Can you work these out from the model? Positions are in its coordinate system, mm. A direction names the side the tool comes from. Round coordinates to 2 decimals unless told otherwise and drop trailing zeros. Loops run counter-clockwise (first coordinate to the right, second up) from the corner with the lowest first, then second, coordinate; pieces in that order, holes last. Notation, with made-up numbers: (49.25, 72.5) -> (74.25, 72.5) arc R21 cw to (74.25, 108.5) -> close; hole circle Ø1 at (22, 65.25). An arc over 180 degrees is marked (long way). Write item = value, one per line.
from build123d import *

# Parameters (mm, degrees)
ESTRUSIONE_ESTRUSIONE1_DEPTH   = 23
FORO_PER_VITE_M3_1_D           = 3.4
FORO_PER_VITE_M3_1_DEPTH       = 34
FORO_PER_VITE_M3_1_CSINK_D     = 3.45
FORO_PER_VITE_M3_1_CSINK_ANGLE = 90
FORO_PER_VITE_M3_1_TIP         = 1.021463052
SCHIZZO5_R                     = 11
ESTRUSIONE_ESTRUSIONE2_DEPTH   = 2
SCHIZZO6_R                     = 2.5
ESTRUSIONE_ESTRUSIONE3_DEPTH   = 18
TAGLIO_ESTRUSIONE1_START       = -17
TAGLIO_ESTRUSIONE1_DEPTH       = 17


with BuildPart() as part:
    # Schizzo1 → Estrusione-Estrusione1 (new body)
    with BuildSketch(Plane(origin=(0, 0, 0), x_dir=(1, 0, 0), z_dir=(0, 1, 0))):
        Polygon((21.15, -17.15), (21.15, 17.15), (17.15, 21.15), (-17.15, 21.15), (-21.15, 17.15), (-21.15, -17.15), (-17.15, -21.15), (17.15, -21.15), align=None)
    extrude(amount=ESTRUSIONE_ESTRUSIONE1_DEPTH)

    # Foro per Vite M3-1
    with Locations(Plane(origin=(0, 0, 0), x_dir=(-1, 0, 0), z_dir=(0, -1, 0))):
        with Locations((-15.5, 15.5), (15.5, 15.5), (15.5, -15.5), (-15.5, -15.5)):
            CounterSinkHole(FORO_PER_VITE_M3_1_D / 2, FORO_PER_VITE_M3_1_CSINK_D / 2, depth=FORO_PER_VITE_M3_1_DEPTH, counter_sink_angle=FORO_PER_VITE_M3_1_CSINK_ANGLE)
            with Locations((0, 0, -(FORO_PER_VITE_M3_1_DEPTH + FORO_PER_VITE_M3_1_TIP / 2))):  # 118° drill point
                Cone(0, FORO_PER_VITE_M3_1_D / 2, FORO_PER_VITE_M3_1_TIP, mode=Mode.SUBTRACT)

    # Schizzo5 → Estrusione-Estrusione2 (add)
    with BuildSketch(Plane(origin=(0, 23, 0), x_dir=(1, 0, 0), z_dir=(0, 1, 0))):
        with Locations(Location((0, 0, 0), (0, 0, 270))):
            Circle(SCHIZZO5_R)
    extrude(amount=ESTRUSIONE_ESTRUSIONE2_DEPTH)

    # Schizzo6 → Estrusione-Estrusione3 (add)
    with BuildSketch(Plane(origin=(0, 25, 0), x_dir=(1, 0, 0), z_dir=(0, 1, 0))):
        with Locations(Location((0, 0, 0), (0, 0, 270))):
            Circle(SCHIZZO6_R)
    extrude(amount=ESTRUSIONE_ESTRUSIONE3_DEPTH)

    # Schizzo7 → Taglio-Estrusione1 (cut)
    with BuildSketch(Plane(origin=(0, 43, 0), x_dir=(1, 0, 0), z_dir=(0, 1, 0)).offset(TAGLIO_ESTRUSIONE1_START)):
        with BuildLine():
            Line((-1.5, 2), (1.5, 2))
            ThreePointArc((1.5, 2), (0, 2.5), (-1.5, 2))
        make_face()
    extrude(amount=TAGLIO_ESTRUSIONE1_DEPTH, mode=Mode.SUBTRACT)


solid = part.part
1. I need wall thicknesses on line 1 (X direction, y = 8.5, z = -15.5); line 2 (Z direction, x = 15, y = 5). Which ranges of each line are inside material? Lowest first, please. Write a range as [from, to].
Entries:
line_1 = [-21.15, -17.2], [-13.8, 13.8], [17.2, 21.15]
line_2 = [-21.15, -17.12], [-13.88, 13.88], [17.12, 21.15]
2. For faces 4 (the flat face through (0, 34, -2)), 5 (the cylindrical face through (0.751, 33.874, 2.385)), 6 (the cylindrical face through (-14.7, 11.7, -14)), which set-ups out of +Z, -Z, +X, -X, +Y, -Y let a thin tool reach every point of the face, with its end or its side?
Entries:
face_4 = -Z, +X, -X, +Y
face_5 = +Y
face_6 = +Y, -Y
3. I'm going to push flat-ended pins straight in: pin 1 (1.5 mm diameter, centred on x = 0, y = 34, fed in from -Z); pin 2 (1 mm diameter, centred on x = 9, z = -3.5, fed in from +Y); pin 3 (5.5 mm diameter, centred on x = 15.5, z = -15.5, fed in from +Y); pin 4 (3 mm diameter, centred on x = -15.5, z = -15.5, fed in from +Y). Where does each tip first touch, or does it pass through?
Entries:
pin_1 = -2
pin_2 = 25
pin_3 = 23
pin_4 = through
4. Suppose I cut it at B-B, the plane z = 15.5. List the corners of the cut face in (x, y) for me (3 decimals).
Entries:
outline = (-21.15, 0) -> (-17.225, 0) -> (-17.2, 0.025) -> (-17.2, 23) -> (-21.15, 23) -> close; (-13.8, 0.025) -> (-13.775, 0) -> (13.775, 0) -> (13.8, 0.025) -> (13.8, 23) -> (-13.8, 23) -> close; (17.2, 0.025) -> (17.225, 0) -> (21.15, 0) -> (21.15, 23) -> (17.2, 23) -> close
5. We'd pull the mould along X, two halves only. Please class faces 1 (the flat face through (0, 11, 21.15)), 2 (the flat face through (-19.2, 11.3, 19.1)), 3 (the cylindrical face through (17.07, 11.67, -14.85)): released by +X, released by -X, zero draft, split by the parting line, or undercut.
Entries:
face_1 = zero draft
face_2 = released by -X
face_3 = undercut
6. Suppose I cut it at A-A, the plane x = -15.5. List the corners of the cut face in (y, z) for me (3 decimals).
Entries:
outline = (0, -21.15) -> (23, -21.15) -> (23, -17.2) -> (0.025, -17.2) -> (0, -17.225) -> close; (0, -13.775) -> (0.025, -13.8) -> (23, -13.8) -> (23, 13.8) -> (0.025, 13.8) -> (0, 13.775) -> close; (0, 17.225) -> (0.025, 17.2) -> (23, 17.2) -> (23, 21.15) -> (0, 21.15) -> close
7. Suppose I cut it at D-D, the plane z = 0. List the corners of the cut face in (x, y) for me, and give its area (3 significant figures).
Entries:
outline = (-21.15, 0) -> (21.15, 0) -> (21.15, 23) -> (11, 23) -> (11, 25) -> (2.5, 25) -> (2.5, 43) -> (-2.5, 43) -> (-2.5, 25) -> (-11, 25) -> (-11, 23) -> (-21.15, 23) -> close
area = 1,110 mm²
8. Suppose I cut it at C-C, the plane y = 10. List the corners of the cut face in (x, z) for me, and give its area (3 significant figures).
Entries:
outline = (-21.15, -17.15) -> (-17.15, -21.15) -> (17.15, -21.15) -> (21.15, -17.15) -> (21.15, 17.15) -> (17.15, 21.15) -> (-17.15, 21.15) -> (-21.15, 17.15) -> close; hole circle Ø3.4 at (-15.5, -15.5); hole circle Ø3.4 at (-15.5, 15.5); hole circle Ø3.4 at (15.5, -15.5); hole circle Ø3.4 at (15.5, 15.5)
area = 1,720 mm²
